Here's how the part is built. I have some questions about the finished solid (model axes, mm). Face numbers are marked on the shaded views. Round coordinates to 2 decimals unless told otherwise and drop trailing zeros. Loops run counter-clockwise (first coordinate to the right, second up) from the corner with the lowest first, then second, coordinate; pieces in that order, holes last. Notation, with made-up numbers: M 55.25,56.5 L 71.25,56.5 A29 cw 71.25,81.5 Z; hole C 30.5,76 d6. An arc over 180 degrees is marked long. Use a Markdown table: item, result.
Autodesk Inventor part; units mm, degrees
ref_plane "YZ Plane" through (0, 0, 0) normal (1, 0, 0) x (0, 1, 0)
ref_plane "XZ Plane" through (0, 0, 0) normal (0, 1, 0) x (-1, 0, 0)
ref_plane "XY Plane" through (0, 0, 0) normal (0, 0, 1) x (1, 0, 0)
sketch "Sketch1" plane through (0, 0, 0) normal (0, 0, 1) x (1, 0, 0)
  line L0 (-27.5, -55) -> (27.5, -55)
  line L1 (27.5, -55) -> (27.5, 55)
  line L2 (27.5, 55) -> (-27.5, 55)
  line L3 (-27.5, 55) -> (-27.5, -55)
  line L4 (-27.5, -55) -> (27.5, 55) construction
  line L5 (27.5, -55) -> (-27.5, 55) construction
  line L6 (0, -77) -> (0, 77)
  line L7 (-38.5, 0) -> (38.5, 0)
  circle A0 centre (-20, 45) radius 2
  circle A1 centre (-20, 5) radius 2
  circle A2 centre (20, 45) radius 2
  circle A3 centre (20, 5) radius 2
  circle A4 centre (-20, -5) radius 2
  circle A5 centre (-20, -45) radius 2
  circle A6 centre (20, -45) radius 2
  circle A7 centre (20, -5) radius 2
  arc A8 (-20, 42.5) -> (-20, 47.5) centre (-20, 45) ccw
  arc A9 (20, 47.5) -> (20, 42.5) centre (20, 45) ccw
  arc A10 (-20, 2.5) -> (-20, 7.5) centre (-20, 5) ccw
  arc A11 (20, 7.5) -> (20, 2.5) centre (20, 5) ccw
  arc A12 (-20, -7.5) -> (-20, -2.5) centre (-20, -5) ccw
  arc A13 (20, -2.5) -> (20, -7.5) centre (20, -5) ccw
  arc A14 (-20, -47.5) -> (-20, -42.5) centre (-20, -45) ccw
  arc A15 (20, -42.5) -> (20, -47.5) centre (20, -45) ccw
  line L8 (-26, -50) -> (24, -50)
  line L9 (24, -50) -> (24, 50)
  line L10 (24, 50) -> (-26, 50)
  line L11 (-26, 50) -> (-26, -50)
  line L12 (-20, 47.5) -> (-26, 47.5)
  line L13 (-20, 42.5) -> (-26, 42.5)
  line L14 (20, 47.5) -> (24, 47.5)
  line L15 (20, 42.5) -> (24, 42.5)
  line L16 (20, 7.5) -> (24, 7.5)
  line L17 (20, 2.5) -> (24, 2.5)
  line L18 (20, -2.5) -> (24, -2.5)
  line L19 (20, -7.5) -> (24, -7.5)
  line L20 (20, -42.5) -> (24, -42.5)
  line L21 (-20, 7.5) -> (-26, 7.5)
  line L22 (-20, 2.5) -> (-26, 2.5)
  line L23 (-20, -2.5) -> (-26, -2.5)
  line L24 (-20, -7.5) -> (-26, -7.5)
  line L25 (-20, -42.5) -> (-26, -42.5)
  line L26 (-20, -47.5) -> (-26, -47.5)
  line L27 (20, -47.5) -> (24, -47.5)
  point P0 (0, 0)
  point P1 (-17.5, 45)
  dimension "d0" = 55
  dimension "d1" = 110
  dimension "d5" = 40
  dimension "d6" = 40
  dimension "d7" = 4
  dimension "d8" = 90
  dimension "d9" = 2.5
  dimension "d10" = 5
  dimension "d12" = 6
  dimension "d13" = 4
extrude "Extrusion1" add sketch "Sketch1" along normal blind 2 contours L3 L7 L11 L8 L6 L0 | L6 L8 L9 L7 L1 L0 | L3 L2 L6 L10 L11 L7 | L7 L9 L10 L6 L2 L1 | L11 L21 A10 L22 | L23 A12 L24 L11 | L11 L25 A14 L26 | L27 A15 L20 L9 | L9 L19 A13 L18 | L17 A11 L16 L9 | L11 L12 A8 L13 | L9 L15 A9 L14
sketch "Sketch3" plane through (0, 0, 0) normal (0, 0, -1) x (-1, 0, 0)
  line L0 (-27.5, 55) -> (27.5, 55)
  line L1 (-16, 55) -> (-24, 55)
  line L2 (-27.5, 55) -> (27.5, 55)
  line L3 (-27.5, -55) -> (-27.5, 55)
  line L4 (27.5, -55) -> (-27.5, -55)
  line L5 (27.5, 55) -> (27.5, -55)
  circle A0 centre (-20, -5) radius 2
  circle A1 centre (-20, 45) radius 2
  circle A2 centre (20, 45) radius 2
  circle A3 centre (-20, 5) radius 2
  circle A4 centre (20, -5) radius 2
  circle A5 centre (-20, -45) radius 2
  circle A6 centre (20, -45) radius 2
  circle A7 centre (20, 5) radius 2
  line L6 (-24, 2.5) -> (-24, -2.5)
  line L7 (-20, 2.5) -> (-24, 2.5)
  arc A8 (-20, 2.5) -> (-20, 7.5) centre (-20, 5) ccw
  line L8 (-24, 7.5) -> (-20, 7.5)
  line L9 (-24, 42.5) -> (-24, 7.5)
  line L10 (-20, 42.5) -> (-24, 42.5)
  arc A9 (-20, 42.5) -> (-20, 47.5) centre (-20, 45) ccw
  line L11 (-24, 47.5) -> (-20, 47.5)
  line L12 (-24, 50) -> (-24, 47.5)
  line L13 (26, 50) -> (-24, 50)
  line L14 (26, 47.5) -> (26, 50)
  line L15 (20, 47.5) -> (26, 47.5)
  arc A10 (20, 47.5) -> (20, 42.5) centre (20, 45) ccw
  line L16 (26, 42.5) -> (20, 42.5)
  line L17 (26, 7.5) -> (26, 42.5)
  line L18 (20, 7.5) -> (26, 7.5)
  arc A11 (20, 7.5) -> (20, 2.5) centre (20, 5) ccw
  line L19 (26, 2.5) -> (20, 2.5)
  line L20 (26, -2.5) -> (26, 2.5)
  line L21 (20, -2.5) -> (26, -2.5)
  arc A12 (20, -2.5) -> (20, -7.5) centre (20, -5) ccw
  line L22 (26, -7.5) -> (20, -7.5)
  line L23 (26, -42.5) -> (26, -7.5)
  line L24 (20, -42.5) -> (26, -42.5)
  arc A13 (20, -42.5) -> (20, -47.5) centre (20, -45) ccw
  line L25 (26, -47.5) -> (20, -47.5)
  line L26 (26, -50) -> (26, -47.5)
  line L27 (-24, -50) -> (26, -50)
  line L28 (-24, -47.5) -> (-24, -50)
  line L29 (-20, -47.5) -> (-24, -47.5)
  arc A14 (-20, -47.5) -> (-20, -42.5) centre (-20, -45) ccw
  line L30 (-24, -42.5) -> (-20, -42.5)
  line L31 (-24, -7.5) -> (-24, -42.5)
  line L32 (-20, -7.5) -> (-24, -7.5)
  arc A15 (-20, -7.5) -> (-20, -2.5) centre (-20, -5) ccw
  line L33 (-24, -2.5) -> (-20, -2.5)
  line L34 (14, 50) -> (22, 50)
  line L35 (22, 55) -> (14, 55)
  line L36 (-27.5, -17) -> (-24, -17)
  line L37 (-24, -17) -> (-24, -9)
  line L38 (-24, -9) -> (-27.5, -9)
  line L39 (-27.5, -9) -> (-27.5, -17)
  line L40 (-27.5, -17) -> (-24, -9) construction
  line L41 (-24, -17) -> (-27.5, -9) construction
  line L42 (-24, 29) -> (-27.5, 29)
  line L43 (-27.5, 29) -> (-27.5, 21)
  line L44 (-27.5, 21) -> (-24, 21)
  line L45 (-24, 21) -> (-24, 29)
  line L46 (-24, 29) -> (-27.5, 21) construction
  line L47 (-27.5, 29) -> (-24, 21) construction
  point P0 (0, 0)
  point P1 (-25.75, -13)
  point P2 (-27.5, -17)
  point P3 (-24, 10.5)
  point P4 (-25.75, 25)
  dimension "d22" = 8
  dimension "d40" = 38
  dimension "d41" = 25
extrude "Extrusion3" add sketch "Sketch3" along normal blind 28 contours L42 L9 L44 L3 | L38 L31 L36 L3
sketch "Sketch5" plane through (0, 0, -28) normal (0, 0, -1) x (-1, 0, 0)
  line L0 (-27.5, -9) -> (-27.5, -17)
  line L1 (-24, 21) -> (-24, 29)
  circle A0 centre (-20, -13) radius 2
  line L2 (-27.5, -9) -> (-27.5, -17)
  arc A1 (-20, -17) -> (-20, -9) centre (-20, -13) ccw
  line L3 (-20, -17) -> (-24, -17)
  line L4 (-24, -9) -> (-20, -9)
  line L5 (-24, -17) -> (-24, -9)
  line L6 (-24, 29) -> (-27.5, 29)
  line L7 (-27.5, 29) -> (-27.5, 21)
  line L8 (-27.5, 21) -> (-24, 21)
  line L9 (-27.5, -17) -> (-24, -17)
  line L10 (-24, -9) -> (-27.5, -9)
  circle A2 centre (-20, 25) radius 2
  arc A3 (-20, 21) -> (-20, 29) centre (-20, 25) ccw
  line L11 (-20, 21) -> (-24, 21)
  line L12 (-24, 29) -> (-27.5, 29)
  line L13 (-24, 29) -> (-20, 29)
  point P0 (0, 0)
  point P1 (-27.5, -13)
  point P2 (-27.5, -13)
  point P3 (-16, -13)
  point P4 (-24, 13)
  point P5 (-24, -17)
  point P6 (-24, -9)
  point P7 (-24, 25)
  point P8 (-16, 25)
  dimension "d36" = 4
  dimension "d37" = 8
extrude "Extrusion5" add sketch "Sketch5" along normal blind 2
properties part number "MTN_PLATE_RETROFIT"
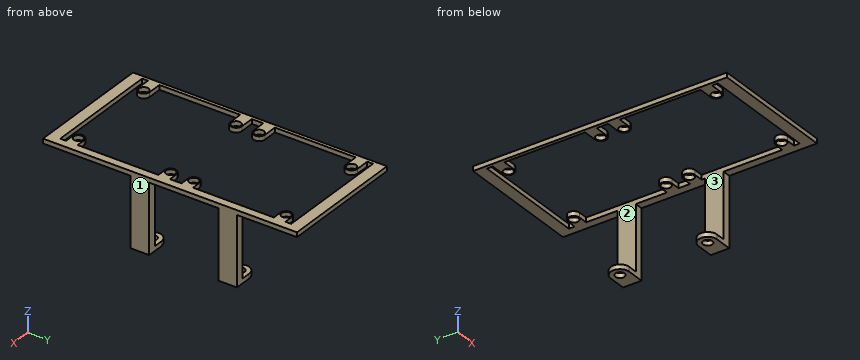
Q1. Imagine slicing it at D-D, the plane y = 25. Please give me the cut outline in (x, z).
Return value:
| item | result |
|---|---|
| outline | M -27.5,0 L -26,0 L -26,2 L -27.5,2 Z; M 16,-30 L 18,-30 L 18,-28 L 16,-28 Z; M 22,-30 L 27.5,-30 L 27.5,2 L 24,2 L 24,-28 L 22,-28 Z |
Q2. Imagine slicing it at C-C, the plane x = -5.5. Please give me the cut outline in (y, z), then the cut area to 3 significant figures.
Return value:
| item | result |
|---|---|
| outline | M -55,0 L -50,0 L -50,2 L -55,2 Z; M 50,0 L 55,0 L 55,2 L 50,2 Z |
| area | 20.0 mm^2 |
Q3. I need wall thicknesses on line 1 (X direction, y = -12.5, z = -23); line 2 (Z direction, x = 23, y = -7). Which ranges of each line are inside material? Lowest first, please. Write a range as from..to.
Return value:
| item | result |
|---|---|
| line 1 | x = 24..27.5 |
| line 2 | z = 0..2 |
Q4. Imagine slicing it at B-B, the plane y = 45. Please give me the cut outline in (x, z).
Return value:
| item | result |
|---|---|
| outline | M -27.5,0 L -22,0 L -22,2 L -27.5,2 Z; M -18,0 L -17.5,0 L -17.5,2 L -18,2 Z; M 17.5,0 L 18,0 L 18,2 L 17.5,2 Z; M 22,0 L 27.5,0 L 27.5,2 L 22,2 Z |
Q5. Will these pins go through, and if not, where does the flat tip stop? P1, Ø6, axis at y = 27.5, z = -14, coming from the -X side; P2, Ø6, axis at x = -21.5, y = -30.5, coming from the -Z side; P3, Ø5, axis at x = 24.5, y = 5, coming from the -Z side.
Return value:
| item | result |
|---|---|
| P1 | stops at x = 24 |
| P2 | passes through |
| P3 | stops at z = 0 |
Q6. Imagine slicing it at A-A, the plane z = -19. Please give me the cut outline in (x, y).
Return value:
| item | result |
|---|---|
| outline | M 24,-17 L 27.5,-17 L 27.5,-9 L 24,-9 Z; M 24,21 L 27.5,21 L 27.5,29 L 24,29 Z |
Q7. We'd pull the mould along Y, two halves only. Please class the marked faces 1, 2 and 3: pulls with the +Y half, pulls with the -Y half, needs draft (parallel to the pull), parting line crosses it, or undercut.
Return value:
| item | result |
|---|---|
| face 1 | needs draft |
| face 2 | undercut |
| face 3 | undercut |
